Verification items for the finished model (mm, model axes). A direction names the side the tool comes from. Coordinates: 2 decimals unless noted, no trailing zeros. Loops run counter-clockwise (first coordinate to the right, second up) from the corner with the lowest first, then second, coordinate; pieces in that order, holes last.
Q1. Access from +Z, -Z, +X, -X, +Y, -Y to the whole of each face (thin tool, end or side, straight path). Record for faces 5 (the face through (-19, 22, 1)), 6 (the face through (-20.93, -21.29, 18.45)), 7 (the face through (8.056, 21.514, -9.554)), 8 (the face through (8.035, -21.486, -9.572)), 9 (the face through (9, -22.5, 7)).
Q2. Sectioned sample at B-B (y = 7). Enter the section's corners in (x, z) (3 decimals).
Q3. Mould release check, pull along Y, two halves, no side actions. Record for faces 1 (the face through (15.636, 15.016, 6.957)), 2 (the face through (-14, 0, -13)), 3 (the face through (-18.95, -21.29, -11.43)), 4 (the face through (-16.364, -14.984, 6.957)): +Y half, -Y half, draft (parallel to the pull), parting line (faces both ways), or undercut.
Q4. Sectioned sample at A-A (z = 0). Enter the section's corners in (x, y) (3 decimals), then the cut area to 3 significant figures.
Q5. Sectioned sample at C-C (z = 15). Enter the section's corners in (x, y).
Q6. Go/stop test with flat-tipped pins: P1, Ø1.5, axis at y = -3, z = -6.5, coming from the -X side; P2, Ø4, axis at y = 7, z = 8, coming from the +X side; P3, Ø16, axis at x = 0, z = 0, coming from the -Y side; P4, Ø4, axis at x = -5, z = -5.5, coming from the +Y side. Record where each tip stops, or that it passes through.
Q7. Material ranges on probe 1 along Y at (x, z) = (-16, 16); probe 2 along X at (y, z) = (15, 14); probe 3 along X at (y, z) = (-3, 0) (3 decimals), recorded low to high.
Q8. Sectioned sample at D-D (x = 0). Enter the section's corners in (y, z) (3 decimals).
```python
from build123d import *

# Parameters (mm, degrees)
F1_DEPTH = 22.5
F2_SIZE  = 2
F4_D     = 4.2
F4_DEPTH = 12
F4_TIP   = 1.2618073


with BuildPart() as f1:
    # F0 (on Front) → F1 (new body, symmetric)
    with BuildSketch(Plane.XZ):
        with BuildLine():
            ThreePointArc((-5, -7.4893274064), (0, 9.005), (5, -7.4893274064))
            Line((5, -7.4893274064), (9.6240033408, -13))
            Line((9.6240033408, -13), (18.5, -13))
            Line((18.5, -13), (20.5, -11))
            Line((20.5, -11), (20.5, 11))
            Line((20.5, 11), (22.5, 13))
            Line((22.5, 13), (22.5, 18))
            Line((22.5, 18), (20.5, 20))
            Line((20.5, 20), (-20.5, 20))
            Line((-20.5, 20), (-22.5, 18))
            Line((-22.5, 18), (-22.5, 13))
            Line((-22.5, 13), (-20.5, 11))
            Line((-20.5, 11), (-20.5, -11))
            Line((-20.5, -11), (-18.5, -13))
            Line((-18.5, -13), (-9.6240033408, -13))
            Line((-9.6240033408, -13), (-5, -7.4893274064))
        make_face()
    extrude(amount=F1_DEPTH, both=True)

    # F2
    f2_edges = [f1.edges().sort_by_distance(p)[0] for p in [
        (0, -22.5, 9.005),
        (7.312002, -22.5, -10.244664),
        (14.062002, -22.5, -13),
        (19.5, -22.5, -12),
        (20.5, -22.5, 0),
        (21.5, -22.5, 12),
        (22.5, -22.5, 15.5),
        (21.5, -22.5, 19),
        (0, -22.5, 20),
        (-21.5, -22.5, 19),
        (-22.5, -22.5, 15.5),
        (-21.5, -22.5, 12),
        (-20.5, -22.5, 0),
        (-19.5, -22.5, -12),
        (-14.062002, -22.5, -13),
        (-7.312002, -22.5, -10.244664),
        (0, 22.5, 9.005),
        (7.312002, 22.5, -10.244664),
        (14.062002, 22.5, -13),
        (19.5, 22.5, -12),
        (20.5, 22.5, 0),
        (21.5, 22.5, 12),
        (22.5, 22.5, 15.5),
        (21.5, 22.5, 19),
        (0, 22.5, 20),
        (-21.5, 22.5, 19),
        (-22.5, 22.5, 15.5),
        (-21.5, 22.5, 12),
        (-20.5, 22.5, 0),
        (-19.5, 22.5, -12),
        (-14.062002, 22.5, -13),
        (-7.312002, 22.5, -10.244664),
    ]]
    chamfer(f2_edges, length=F2_SIZE)

    # F4
    with Locations(Plane.XY.offset(20)):
        with Locations((-16, 15), (16, 15), (16, -15), (-16, -15)):
            Hole(F4_D / 2, depth=F4_DEPTH)
            with Locations((0, 0, -(F4_DEPTH + F4_TIP / 2))):  # 118° drill point
                Cone(0, F4_D / 2, F4_TIP, mode=Mode.SUBTRACT)


solid = f1.part
```
Geometry check:
1. face 5: -Z, -X, +Y
1. face 6: +Z, -X, -Y
1. face 7: -Z, +Y
1. face 8: -Z, -Y
1. face 9: +Z, -Z, +X, -X, -Y
2. outline: (-22.5, 13) - (-20.5, 11) - (-20.5, -11) - (-18.5, -13) - (-9.624, -13) - (-5, -7.489) arc R9.005 cw (long way) to (5, -7.489) - (9.624, -13) - (18.5, -13) - (20.5, -11) - (20.5, 11) - (22.5, 13) - (22.5, 18) - (20.5, 20) - (-20.5, 20) - (-22.5, 18) - close
3. face 1: undercut
3. face 2: draft
3. face 3: -Y half
3. face 4: undercut
4. outline: (-20.5, -20.5) - (-18.5, -22.5) - (-11.005, -22.5) - (-9.005, -20.5) - (-9.005, 20.5) - (-11.005, 22.5) - (-18.5, 22.5) - (-20.5, 20.5) - close; (9.005, -20.5) - (11.005, -22.5) - (18.5, -22.5) - (20.5, -20.5) - (20.5, 20.5) - (18.5, 22.5) - (11.005, 22.5) - (9.005, 20.5) - close
4. area: 1,020 mm2
5. outline: (-22.5, -20.5) - (-20.5, -22.5) - (20.5, -22.5) - (22.5, -20.5) - (22.5, 20.5) - (20.5, 22.5) - (-20.5, 22.5) - (-22.5, 20.5) - close; hole circle Ø4.2 at (-16, -15); hole circle Ø4.2 at (-16, 15); hole circle Ø4.2 at (16, -15); hole circle Ø4.2 at (16, 15)
6. P1: stops at x = -20.5
6. P2: stops at x = 20.5
6. P3: passes through
6. P4: stops at y = 20.93
7. probe 1: y = -22.5 to -17.1, -12.9 to 12.9, 17.1 to 22.5
7. probe 2: x = -22.5 to -18.1, -13.9 to 13.9, 18.1 to 22.5
7. probe 3: x = -20.5 to -9.005, 9.005 to 20.5
8. outline: (-22.5, 11.005) - (-20.5, 9.005) - (20.5, 9.005) - (22.5, 11.005) - (22.5, 18) - (20.5, 20) - (-20.5, 20) - (-22.5, 18) - close
